Autodesk Inventor part; units mm, degrees
ref_plane "YZ Plane" through (0, 0, 0) normal (1, 0, 0) x (0, 1, 0)
ref_plane "XZ Plane" through (0, 0, 0) normal (0, 1, 0) x (-1, 0, 0)
ref_plane "XY Plane" through (0, 0, 0) normal (0, 0, 1) x (1, 0, 0)
sketch "Sketch1" plane through (0, 0, 0) normal (0, 1, 0) x (-1, 0, 0)
  line L0 (0, 0) -> (37, 0)
  line L1 (37, 0) -> (37, -119)
  line L2 (37, -119) -> (0, -119)
  line L3 (0, -119) -> (0, 0)
  dimension "d0" = 37
  dimension "d1" = 119
extrude "Extrusion1" add sketch "Sketch1" along normal blind 2
sketch "Sketch3" plane through (0, 0, 0) normal (0, -1, 0) x (1, 0, 0)
  line L0 (0, 0) -> (-16.5, 0)
  line L1 (-37, 0) -> (0, 0)
  line L2 (-19, 0) -> (-19, -2)
  arc A0 (-21.5, -2) -> (-16.5, -2) centre (-19, -2) ccw
  line L3 (0, 0) -> (0, -119)
  line L4 (0, -119) -> (-19, -119)
  line L5 (0, -119) -> (-37, -119)
  line L6 (-19, -119) -> (-19, -117)
  arc A1 (-16.5, -117) -> (-21.5, -117) centre (-19, -117) ccw
  line L7 (-16.5, -117) -> (-16.5, -119)
  line L8 (-21.5, -117) -> (-21.5, -119)
  line L9 (-21.5, -119) -> (-16.5, -119)
  line L10 (-21.5, -2) -> (-21.5, 0)
  line L11 (-16.5, -2) -> (-16.5, 0)
  line L12 (-21.5, 0) -> (-16.5, 0)
  dimension "d14" = 19
  dimension "d15" = 2
  dimension "d16" = 5
  dimension "d17" = 19
  dimension "d18" = 2
  dimension "d19" = 5
extrude "Extrusion3" cut sketch "Sketch3" against normal blind 2
sketch "Sketch4" plane through (0, 2, 0) normal (0, 1, 0) x (1, 0, 0)
  line L0 (0, 119) -> (0, 0)
  line L1 (0, 0) -> (0, 10)
  line L2 (0, 10) -> (-6, 10)
  line L3 (-32, 10) -> (-32, 105)
  line L4 (-6, 105) -> (-6, 10)
  line L5 (-6, 10) -> (-12.1, 10)
  line L6 (-6, 105) -> (-10.2, 105)
  line L7 (-10.2, 105) -> (-12.1, 105)
  line L8 (-12.5, 105) -> (-12.5, 107.7)
  line L9 (-12.5, 107.7) -> (-10.2, 107.7)
  line L10 (-10.2, 107.7) -> (-10.2, 105)
  line L11 (-6, 10) -> (-8, 10)
  line L12 (-8, 10) -> (-8, 105)
  line L13 (-12.5, 105) -> (-12.5, 103)
  line L14 (-12.5, 103) -> (-10, 103)
  line L15 (-10, 103) -> (-10, 12)
  line L16 (-6, 10) -> (-12.1, 10)
  line L17 (-15.4, 10) -> (-32, 10)
  line L18 (-32, 105) -> (-12.5, 105)
  line L19 (-10.2, 105) -> (-6, 105)
  line L20 (-10, 12) -> (-12.5, 12)
  line L21 (-12.5, 12) -> (-12.5, 10)
  line L22 (-12.5, 10) -> (-12.5, 7.3)
  line L23 (-12.5, 7.3) -> (-10.2, 7.3)
  line L24 (-10.2, 7.3) -> (-10.2, 10)
  line L25 (-15.4, 10) -> (-12.5, 10)
  point P0 (-19, 2)
  dimension "d59" = 10
  dimension "d60" = 6
  dimension "d61" = 26
  dimension "d62" = 95
  dimension "d66" = 4.2
  dimension "d67" = 2.3
  dimension "d73" = 2
  dimension "d76" = 2.5
  dimension "d101" = 2.5
  dimension "d102" = 2.7
  dimension "d103" = 4.5
  dimension "d106" = 2
  dimension "d107" = 2.7
  dimension "d108" = 2
  dimension "d109" = 2
  dimension "d110" = 2
extrude "Extrusion7" add sketch "Sketch4" against normal blind 92 contours L8 L9 L10 L6 L12 L5 L24 L23 L22 L21 L20 L15 L14 L13 | L6 L4 L5 L12
sketch "Sketch6" plane through (-10, -90, -103) normal (-1, 0, 0) x (0, 0, 1)
  line L0 (103, 92) -> (-16, 92)
  line L1 (-4.7, 92) -> (60.3, 92)
  line L2 (60.3, 92) -> (60.3, 66.128)
  circle A0 centre (60.3, 66.128) radius 1.375
  line L3 (-4.7, 90) -> (-4.7, 0)
  line L4 (60.3, 66.128) -> (60.3, 8.128)
  circle A1 centre (60.3, 8.128) radius 1.375
  line L5 (60.3, 8.128) -> (11.3, 8.128)
  circle A2 centre (11.3, 8.128) radius 1.375
  line L6 (11.3, 8.128) -> (11.3, 66.128)
  circle A3 centre (11.3, 66.128) radius 1.375
  point P0 (103, 90)
  dimension "d16" = 5
  dimension "d80" = 65
  dimension "d81" = 25.872
  dimension "d82" = 2.75
  dimension "d83" = 65
  dimension "d87" = 58
  dimension "d88" = 2.75
  dimension "d89" = 49
  dimension "d90" = 2.75
  dimension "d91" = 2.75
extrude "Extrusion8" cut sketch "Sketch6" against normal blind 2
sketch "Sketch7" plane through (0, 0, 0) normal (0, -1, 0) x (1, 0, 0)
  line L0 (-10, -103) -> (-10, -12)
  line L1 (-10, -103) -> (-10, -41)
  line L2 (-10, -41) -> (-12.9, -41)
  line L3 (-12.9, -41) -> (-28.9, -41)
  line L4 (-28.9, -41) -> (-28.9, -95)
  line L5 (-28.9, -95) -> (-12.9, -95)
  line L6 (-12.9, -95) -> (-12.9, -41)
  point P0 (0, 0)
  dimension "d94" = 62
  dimension "d95" = 2.9
  dimension "d96" = 16
  dimension "d97" = 54
extrude "Extrusion9" cut sketch "Sketch7" against normal blind 2
sketch "Sketch8" plane through (-6, -90, -10) normal (1, 0, 0) x (0, 0, -1)
  line L0 (0, 90) -> (0, 0)
  line L1 (95, 90) -> (95, 0)
  line L2 (0, 0) -> (95, 0)
  line L3 (95, 0) -> (95, 90)
  line L4 (95, 90) -> (0, 90)
  line L5 (0, 90) -> (0, 0)
  point P0 (-10, 90)
extrude "Extrusion10" cut sketch "Sketch8" against normal blind 2
properties part number "Slot"
The model under review builds one solid part; all positions refer to its coordinate system, in mm. A direction names the side the tool comes from. Round coordinates to 2 decimals unless told otherwise and drop trailing zeros. Write each loop counter-clockwise with the first axis right and the second up, starting at its lowest first coordinate (ties: lowest second). Pieces come first, ordered by that corner, then holes. Notation, with made-up numbers: M -9,58 L 46,58 A24 cw 46,85 Z; hole C 53,9 d4. An arc over 180 degrees is marked long. Use CSV: the item, a comma, the result in double quotes. Start each with the question number.
(1) We need section D-D, the plane y = -77. State the section outline as (x, z) points.
(2) For line 1 along Y through (x, z) = (-9.45, -91.7); line 2 along Y through (x, z) = (-9, -42); line 3 along X through (y, z) = (-20, -79.5), list the stretches that pass through material, from the lowest coordinate up.
(3) We need section A-A, the plane z = -53. State the section outline as (x, y) points, then the cut area to 3 significant figures.
(4) We need section B-B, the plane x = -19. State the section outline as (y, z) points.
(5) Clearance check with flat-ended pins moving along their axes: P1, Ø4, axis at y = -25.5, z = -9, coming from the -X side; P2, Ø0.7, axis at x = -11.5, y = -58, coming from the +Z side; P3, Ø11, axis at x = -19.5, z = -41, coming from the -Y side; P4, Ø3, axis at x = -26.5, z = -47.5, coming from the +Y side. State where each tip first meets the part, or that it passes through.
(6) Tool access review of faces 1 (the face through (-11, -44, -103)), 2 (the face through (-6, 0, -59)), 3 (the face through (-8, -44, -57)), 4 (the face through (-10.2, -44, -9)): name each direction out of +Z, -Z, +X, -X, +Y, -Y from which nothing blocks a thin tool from reaching the whole face with its end or side.
(7) We need section C-C, the plane z = -36.5. State the section outline as (x, y) points.
(8) The part is to be moulded in two halves that separate along X. For faces 5 (the face through (-18.9, 1, -114.5)), 6 (the face through (-9.014, -23.812, -93.074)), 7 (the face through (-10.2, -44, -106)), say which applies: +X half, -X half, draft (parallel to the pull), parting line (faces both ways), or undercut.
Findings:
1,outline,"M -12.5,-107.7 L -10.2,-107.7 L -10.2,-105 L -8,-105 L -8,-10 L -10.2,-10 L -10.2,-7.3 L -12.5,-7.3 L -12.5,-12 L -10,-12 L -10,-103 L -12.5,-103 Z"
2,line 1,"-90 to -83.25, -80.5 to -25.25, -22.5 to 2"
2,line 2,"-90 to -83.06, -80.69 to -25.06, -22.69 to 2"
2,line 3,"-10 to -8"
3,outline,"M -37,0 L -28.9,0 L -28.9,2 L -37,2 Z; M -12.9,0 L -10,0 L -10,-90 L -8,-90 L -8,0 L 0,0 L 0,2 L -12.9,2 Z"
3,area,"222 mm^2"
4,outline,"M 0,-114.5 L 2,-114.5 L 2,-95 L 0,-95 Z; M 0,-41 L 2,-41 L 2,-4.5 L 0,-4.5 Z"
5,P1,"x = -12.5"
5,P2,"z = -7.3"
5,P3,"y = 0"
5,P4,"through"
6,face 1,"-X, -Y"
6,face 2,"-Y"
6,face 3,"+Z, -Z, +X, -Y"
6,face 4,"+Z, +X, -Y"
7,outline,"M -37,0 L -10,0 L -10,-90 L -8,-90 L -8,0 L 0,0 L 0,2 L -37,2 Z"
8,face 5,"undercut"
8,face 6,"draft"
8,face 7,"+X half"
